```python
from build123d import *

# Parameters (mm, degrees)
SKETCH1_R                = 19
SKETCH1_R_2              = 16
BOSS_EXTRUDE1_DEPTH      = 40
SKETCH2_W                = 60
SKETCH2_H                = 40
SKETCH2_R                = 19
BOSS_EXTRUDE2_DEPTH      = 3
SKETCH4_R                = 2.5
CUT_EXTRUDE1_DEPTH       = 54.851648071
BOSS_EXTRUDE3_DEPTH      = 16
BOSS_EXTRUDE3_DEPTH_BACK = 16
SKETCH6_R                = 16
SKETCH6_R_2              = 10


with BuildPart() as part:
    # Sketch1 → Boss-Extrude1 (new body)
    with BuildSketch(Plane.XY):
        Circle(SKETCH1_R)
        Circle(SKETCH1_R_2, mode=Mode.SUBTRACT)
    extrude(amount=BOSS_EXTRUDE1_DEPTH)

    # Sketch2 → Boss-Extrude2 (add)
    with BuildSketch(Plane(origin=(0, 0, 0), x_dir=(-1, 0, 0), z_dir=(0, 0, -1))):
        Rectangle(SKETCH2_W, SKETCH2_H)
        Circle(SKETCH2_R, mode=Mode.SUBTRACT)
    boss_extrude2 = extrude(amount=-BOSS_EXTRUDE2_DEPTH)

    # Mirror1: Boss-Extrude2 across plane
    add(boss_extrude2.mirror(Plane.XY.offset(20)))

    # Sketch4 → Cut-Extrude1 (cut, through all)
    with BuildSketch(Plane(origin=(0, 0, 0), x_dir=(-1, 0, 0), z_dir=(0, 0, -1))):
        with Locations((-25, 14.38623609)):
            Circle(SKETCH4_R)
        with Locations((25, 14.38623609)):
            Circle(SKETCH4_R)
        with Locations((-25, -13.739663681)):
            Circle(SKETCH4_R)
        with Locations((25, -13.739663681)):
            Circle(SKETCH4_R)
    extrude(amount=-CUT_EXTRUDE1_DEPTH, mode=Mode.SUBTRACT)

    # Sketch6 → Boss-Extrude3 (add, two sides: drawn at the far end of the back side and taken through both)
    with BuildSketch(Plane.XY.offset(20).offset(-BOSS_EXTRUDE3_DEPTH_BACK)):
        Circle(SKETCH6_R)
        Circle(SKETCH6_R_2, mode=Mode.SUBTRACT)
    extrude(amount=BOSS_EXTRUDE3_DEPTH + BOSS_EXTRUDE3_DEPTH_BACK)


solid = part.part
```
Model file for the job. Use its own axes, mm. A direction names the side the tool comes from. Round coordinates to 2 decimals unless told otherwise and drop trailing zeros. Loops run counter-clockwise (first coordinate to the right, second up) from the corner with the lowest first, then second, coordinate; pieces in that order, holes last. Notation, with made-up numbers: M -20,6 L -2,6 A33 cw -2,41 Z; hole C 35.5,11 d8. An arc over 180 degrees is marked long. Put each result on its own line as item: value. Start each with the question number.
Item 1: Cut at B-B (x = 0). List the corners of the cut face in (y, z).
Item 2: Drop flat-ended pins along their axis: P1, Ø5, axis at y = 10, z = 26, coming from the -X side; P2, Ø12, axis at x = 13.5, y = 7.5, coming from the -Z side; P3, Ø5, axis at y = -4.5, z = 26, coming from the +X side; P4, Ø3, axis at y = 5.5, z = 26.5, coming from the -X side. Give the stop position or say it passes through.
Item 3: Drill centre lines: line 1 along Y through (x, z) = (25, 1); line 2 along Z through (x, y) = (-13, 14.5); line 3 along Z through (x, y) = (13, -8.5). Where is each one in solid material? Low to high.
Item 4: Cut at A-A (y = 0). List the corners of the cut face in (x, z), then the cut area to 3 significant figures.
Item 5: Mould opens along Z. For faces 1 (the face through (10.4, 0.2, 36)), 2 (the face through (14, 9, 0)), 3 (the face through (26.984, -15.261, 38.479)), 4 (the face through (7, 18, 37)) say: released by +Z, released by -Z, zero draft, split by the parting line, or undercut.
Item 6: 3-axis set-ups, long thin cutter, end or side, ignore diameter. For faces 5 (the face through (26.84, 16.08, 38.48)), 6 (the face through (-3.47, -15.62, 37.97)), 7 (the face through (-30, 0, 39)), 8 (the face through (8.767, -16.856, 19.762)), 9 (the face through (10.4, 0.2, 4)): which of +Z, -Z, +X, -X, +Y, -Y reach the whole face in a straight line?
Item 7: Cut at C-C (x = 25). List the corners of the cut face in (y, z).
Item 8: Cut at D-D (z = 28.5). List the corners of the cut face in (x, y), then the cut area to 3 significant figures.
Answer block:
1. outline: M -20,0 L -16,0 L -16,4 L -10,4 L -10,36 L -16,36 L -16,40 L -20,40 L -20,37 L -19,37 L -19,3 L -20,3 Z; M 10,4 L 16,4 L 16,0 L 20,0 L 20,3 L 19,3 L 19,37 L 20,37 L 20,40 L 16,40 L 16,36 L 10,36 Z
2. P1: x = -17.46
2. P2: z = 0
2. P3: x = 18.89
2. P4: x = -18.57
3. line 1: -20 to -16.24, -11.24 to 11.89, 16.89 to 20
3. line 2: 0 to 3, 37 to 40
3. line 3: 4 to 36
4. outline: M -30,0 L -16,0 L -16,4 L -10,4 L -10,36 L -16,36 L -16,40 L -30,40 L -30,37 L -19,37 L -19,3 L -30,3 Z; M 10,4 L 16,4 L 16,0 L 30,0 L 30,3 L 19,3 L 19,37 L 30,37 L 30,40 L 16,40 L 16,36 L 10,36 Z
4. area: 756 mm2
5. face 1: released by +Z
5. face 2: released by -Z
5. face 3: zero draft
5. face 4: undercut
6. face 5: +Z, -Z
6. face 6: +Z
6. face 7: +Z, -Z, -X, +Y, -Y
6. face 8: none
6. face 9: -Z
7. outline: M -20,0 L -16.24,0 L -16.24,3 L -20,3 Z; M -20,37 L -16.24,37 L -16.24,40 L -20,40 Z; M -11.24,0 L 11.89,0 L 11.89,3 L -11.24,3 Z; M -11.24,37 L 11.89,37 L 11.89,40 L -11.24,40 Z; M 16.89,0 L 20,0 L 20,3 L 16.89,3 Z; M 16.89,37 L 20,37 L 20,40 L 16.89,40 Z
8. outline: C 0,0 d38; hole C 0,0 d20
8. area: 820 mm2
